Geometry: see drawing. Coordinates: mm, zero at the bounding-box minimum. A direction names the side the tool comes from. Round coordinates to 2 decimals unless told otherwise and drop trailing zeros. Loops run counter-clockwise (first coordinate to the right, second up) from the corner with the lowest first, then second, coordinate; pieces in that order, holes last.
(1) Access query for the marked faces 5, 6, 7 and 8. Directions: +Z, -Z, +X, -X, +Y, -Y. A direction counts if a zero-diameter tool reaches every point of the face in a straight line with its end or side. Return the directions, or none.
(2) Cut plane B-B, the plane x = 12.7. Output: boundary loops of the cut face in (y, z) (1 decimal).
(3) First-contact query: pin 1 Ø7.5 at (x, z) = (7, 29) entering from +Y (1 decimal); pin 2 Ø5 at (x, y) = (6, 10.5) entering from -Z; pin 3 Ø5 at (x, y) = (14.5, 8) entering from +Z. Flat tips, straight axial feed; report the tip coordinate or a pass-through.
(4) Line query: line 1 (Z direction, x = 15.5, y = 22.75) (1 decimal); line 2 (Z direction, x = 1.5, y = 3.5) (1 decimal). Output: solid intervals per line, ascending.
(5) Cut plane A-A, the plane z = 24. Output: boundary loops of the cut face in (x, y) (1 decimal).
(6) Draft query along Z for the marked faces 1, 2, 3 and 4. Return one class per face: released by +Z, released by -Z, zero draft, split by the parting line, or undercut.
(7) Cut plane C-C, the plane x = 6.35. Output: boundary loops of the cut face in (y, z) (1 decimal).
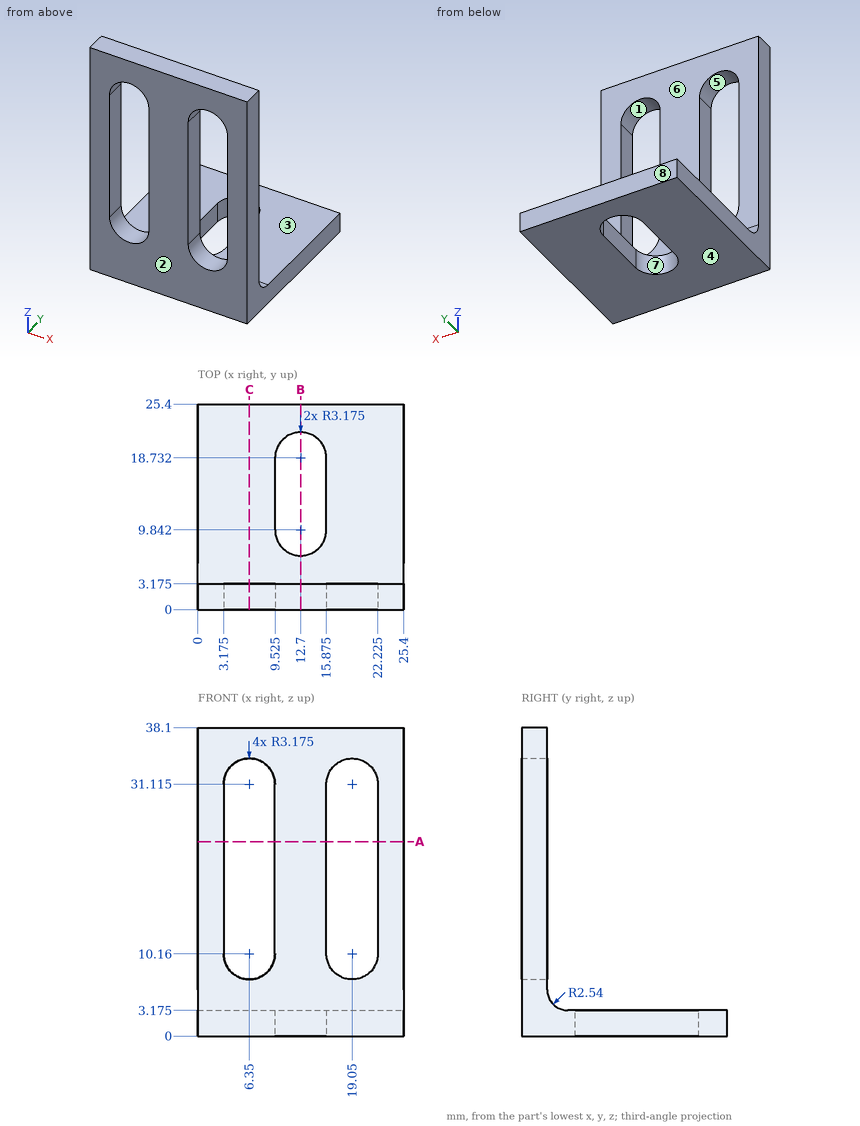
Reported:
1. face 5: +Y, -Y
1. face 6: +Z, +X, -X, +Y
1. face 7: +Z, -Z
1. face 8: +Z, -Z, +X, -X, +Y
2. outline: (0, 0) - (6.7, 0) - (6.7, 3.2) - (5.7, 3.2) arc R2.5 cw to (3.2, 5.7) - (3.2, 38.1) - (0, 38.1) - close; (21.9, 0) - (25.4, 0) - (25.4, 3.2) - (21.9, 3.2) - close
3. pin 1: stops at y = 3.2
3. pin 2: stops at z = 0
3. pin 3: stops at z = 3.18
4. line 1: z = 0 to 3.2
4. line 2: z = 0 to 4.5
5. outline: (0, 0) - (3.2, 0) - (3.2, 3.2) - (0, 3.2) - close; (9.5, 0) - (15.9, 0) - (15.9, 3.2) - (9.5, 3.2) - close; (22.2, 0) - (25.4, 0) - (25.4, 3.2) - (22.2, 3.2) - close
6. face 1: undercut
6. face 2: zero draft
6. face 3: released by +Z
6. face 4: released by -Z
7. outline: (0, 0) - (25.4, 0) - (25.4, 3.2) - (5.7, 3.2) arc R2.5 cw to (3.2, 5.7) - (3.2, 7) - (0, 7) - close; (0, 34.3) - (3.2, 34.3) - (3.2, 38.1) - (0, 38.1) - close
